```python
from build123d import *

# Parameters (mm, degrees)
BOSS_EXTRUDE1_DEPTH = 3
CUT_EXTRUDE2_REACH  = 34.033
SKETCH2_R           = 1.85
CHAMFER2_SIZE       = 0.5


with BuildPart() as part:
    # Sketch1 → Boss-Extrude1 (new, symmetric)
    with BuildSketch(Plane.XY):
        with BuildLine():
            Line((-31.021944793, 0), (-22.806809681, 0))
            ThreePointArc((-22.806809681, 0), (-22.205768917, 0.248959236), (-21.956809681, 0.85))
            Line((-21.956809681, 0.85), (-21.956809681, 1.36849254))
            ThreePointArc((-21.956809681, 1.36849254), (-21.965643691, 1.490720925), (-21.9919621, 1.610408683))
            ThreePointArc((-21.9919621, 1.610408683), (-19.163961672, 5.4), (-16.335961244, 1.610408683))
            ThreePointArc((-16.335961244, 1.610408683), (-16.362279653, 1.490720925), (-16.371113663, 1.36849254))
            Line((-16.371113663, 1.36849254), (-16.371113663, 0.85))
            ThreePointArc((-16.371113663, 0.85), (-16.122154427, 0.248959236), (-15.521113663, 0))
            Line((-15.521113663, 0), (3.236038328, 0))
            ThreePointArc((3.236038328, 0), (3.731013075, 0.205025253), (3.936038328, 0.7))
            Line((3.936038328, 0.7), (3.936038328, 0.937652462))
            ThreePointArc((3.936038328, 0.937652462), (3.932728617, 1.005642472), (3.922830781, 1.072989547))
            ThreePointArc((3.922830781, 1.072989547), (5.836038328, 3.4), (7.749245875, 1.072989547))
            ThreePointArc((7.749245875, 1.072989547), (7.739348039, 1.005642472), (7.736038328, 0.937652462))
            Line((7.736038328, 0.937652462), (7.736038328, 0.7))
            ThreePointArc((7.736038328, 0.7), (7.941063581, 0.205025253), (8.436038328, 0))
            Line((8.436038328, 0), (18.686038328, 0))
            ThreePointArc((18.686038328, 0), (19.039591719, 0.146446609), (19.186038328, 0.5))
            Line((19.186038328, 0.5), (19.186038328, 0.733631047))
            ThreePointArc((19.186038328, 0.733631047), (19.183189302, 0.786931226), (19.174674692, 0.839623991))
            ThreePointArc((19.174674692, 0.839623991), (20.836038328, 2.9), (22.497401964, 0.839623991))
            ThreePointArc((22.497401964, 0.839623991), (22.488887354, 0.786931226), (22.486038328, 0.733631047))
            Line((22.486038328, 0.733631047), (22.486038328, 0.5))
            ThreePointArc((22.486038328, 0.5), (22.632484937, 0.146446609), (22.986038328, 0))
            Line((22.986038328, 0), (31.021944793, 0))
            Line((31.021944793, 0), (31.021944793, 1.5))
            Line((31.021944793, 1.5), (24.021944793, 1.5))
            ThreePointArc((24.021944793, 1.5), (20.836038328, 4.4), (17.650131864, 1.5))
            Line((17.650131864, 1.5), (9.28567599, 1.5))
            ThreePointArc((9.28567599, 1.5), (5.836038328, 4.9), (2.386400666, 1.5))
            Line((2.386400666, 1.5), (-14.305978551, 1.5))
            ThreePointArc((-14.305978551, 1.5), (-19.163961672, 7.4), (-24.021944793, 1.5))
            Line((-24.021944793, 1.5), (-31.021944793, 1.5))
            Line((-31.021944793, 1.5), (-31.021944793, 0))
        make_face()
    extrude(amount=BOSS_EXTRUDE1_DEPTH, both=True)

    # Sketch2 → Cut-Extrude2 (cut, up to next)
    with BuildSketch(Plane(origin=(0, 0, 0), x_dir=(1, 0, 0), z_dir=(0, 1, 0)), mode=Mode.PRIVATE) as cut_extrude2_sk1:
        with Locations(Location((-27.521944793, 0, 0), (0, 0, 90))):
            Circle(SKETCH2_R)
    cut_extrude2_tool1 = extrude(cut_extrude2_sk1.sketch, amount=CUT_EXTRUDE2_REACH, mode=Mode.PRIVATE) & part.part
    # Sketch2 → Cut-Extrude2 (cut, up to next)
    with BuildSketch(Plane(origin=(0, 0, 0), x_dir=(1, 0, 0), z_dir=(0, 1, 0)), mode=Mode.PRIVATE) as cut_extrude2_sk2:
        with Locations(Location((-5.659788943, 0, 0), (0, 0, 90))):
            Circle(SKETCH2_R)
    cut_extrude2_tool2 = extrude(cut_extrude2_sk2.sketch, amount=CUT_EXTRUDE2_REACH, mode=Mode.PRIVATE) & part.part
    # Sketch2 → Cut-Extrude2 (cut, up to next)
    with BuildSketch(Plane(origin=(0, 0, 0), x_dir=(1, 0, 0), z_dir=(0, 1, 0)), mode=Mode.PRIVATE) as cut_extrude2_sk3:
        with Locations(Location((27.521944793, 0, 0), (0, 0, 90))):
            Circle(SKETCH2_R)
    cut_extrude2_tool3 = extrude(cut_extrude2_sk3.sketch, amount=CUT_EXTRUDE2_REACH, mode=Mode.PRIVATE) & part.part
    # Sketch2 → Cut-Extrude2 (cut, up to next)
    with BuildSketch(Plane(origin=(0, 0, 0), x_dir=(1, 0, 0), z_dir=(0, 1, 0)), mode=Mode.PRIVATE) as cut_extrude2_sk4:
        with Locations(Location((13.467903927, 0, 0), (0, 0, 90))):
            Circle(SKETCH2_R)
    cut_extrude2_tool4 = extrude(cut_extrude2_sk4.sketch, amount=CUT_EXTRUDE2_REACH, mode=Mode.PRIVATE) & part.part
    add(cut_extrude2_tool1.solids().sort_by_distance((-27.521945, 0, 0))[0], mode=Mode.SUBTRACT)
    add(cut_extrude2_tool2.solids().sort_by_distance((-5.659789, 0, 0))[0], mode=Mode.SUBTRACT)
    add(cut_extrude2_tool3.solids().sort_by_distance((27.521945, 0, 0))[0], mode=Mode.SUBTRACT)
    add(cut_extrude2_tool4.solids().sort_by_distance((13.467904, 0, 0))[0], mode=Mode.SUBTRACT)

    # Chamfer2
    chamfer2_edges = [part.edges().sort_by_distance(p)[0] for p in [
        (-27.521944793, 1.5, 1.85),
        (-5.659788943, 1.5, 1.85),
        (13.467903927, 1.5, 1.85),
        (27.521944793, 1.5, 1.85),
    ]]
    chamfer(chamfer2_edges, length=CHAMFER2_SIZE)


solid = part.part
```
Here's how the part is built. I have some questions about the finished solid (model axes, mm). A direction names the side the tool comes from. Give positions to 0.01 mm unless a question says otherwise; leave off trailing zeros. Write each loop counter-clockwise with the first axis right and the second up, starting at its lowest first coordinate (ties: lowest second). Pieces come first, ordered by that corner, then holes. Notation, with made-up numbers: M -1.75,14.25 L 34.25,14.25 A11 ccw 34.25,32.25 Z; hole C -29.75,64.5 d11. An arc over 180 degrees is marked long. Put each result on its own line as item: value. Start each with the question number.
Item 1: On a 3-axis mill with a long thin cutter (end or side, diameter ignored), from which of +Z, -Z, +X, -X, +Y, -Y can I reach the whole of each face in a straight line? I mean faces 4 (the cylindrical face through (-7.5, 0.5, 0.2)), 5 (the flat face through (30, 1.5, 1)). Say none if no direction works.
Item 2: If we section it at B-B, the plane x = 20.5: Write out the boundary of the cut face in (y, z), then the cut area to 3 significant figures.
Item 3: I need wall thicknesses on L1, parallel to X at y = 2.25, z = -0.25; L2, parallel to X at y = 1.75, z = 2; L3, parallel to Y at x = 10.5, z = 0.8. Which ranges of each line are inside material? Lowest first, please. Write a range as from..to.
Item 4: If we section it at A-A, the plane z = 0: Count the separate pieces of the cut face and the enclosed holes in it, then the cut area to 3 significant figures.
Item 5: Thinking about a two-plate mould opening in X: for faces 1 (the cylindrical face through (-29.356, 0.493, 0.241)), 2 (the flat face through (-31.022, 1, 0)), 3 (the flat face through (26.05, 0, 1.38)), which applies, +X half, -X half, draft (parallel to the pull), parting line (faces both ways), or undercut?
Item 6: If we section it at C-C, the plane y = 6.75: Write out the boundary of the cut face in (x, z), then the cut area to 3 significant figures.
Item 7: Will these pins go through, and if not, where does the flat tip stop? pin 1 (1.5 mm diameter, centred on x = 23.5, y = 5, fed in from +Z); pin 2 (1.5 mm diameter, centred on x = -4, z = 0, fed in from +Y); pin 3 (1.8 mm diameter, centred on x = -28, z = 1, fed in from +Y).
Values:
1. face 4: +Y, -Y
1. face 5: +Z, -Z, +X, +Y
2. outline: M 2.87,-3 L 4.38,-3 L 4.38,3 L 2.87,3 Z
2. area: 9.10 mm²
3. L1: -24.11..-22.11, -16.22..-14.22, 2.48..4.06, 7.61..9.19, 17.81..19.5, 22.17..23.86
3. L2: -24.06..-22.03, -16.3..-14.26, 2.4..3.91, 7.76..9.27, 17.68..19.23, 22.44..23.99
3. L3: 0..1.5
4. separate pieces: 5
4. enclosed holes: 0
4. area: 102 mm²
5. face 1: undercut
5. face 2: -X half
5. face 3: draft
6. outline: M -21.62,-3 L -16.71,-3 L -16.71,3 L -21.62,3 Z
6. area: 29.4 mm²
7. pin 1: through
7. pin 2: y = 1.5
7. pin 3: y = 1.16
